from build123d import *

# Parameters (mm, degrees)
F1_DEPTH = 130
F2_W     = 50.8
F2_H     = 25.4
F3_DEPTH = 79.5
F4_W     = 12
F4_H     = 50.7057624385
F4_H_2   = 69.7820825055
F4_H_3   = 69.8881107867
F4_H_4   = 52.3517530859
F5_DEPTH = 47.4990536315


# Not quite as in the source:
# - ends of sketch curves that miss each other by under 0.0002 mm in the source are joined
# - a feature names something its author has since deleted; it is built from what else it names


with BuildPart() as f1:
    # F0 (on Right) → F1 (new body)
    with BuildSketch(Plane.YZ):
        with BuildLine():
            Line((62.1368927236, 13.271021442), (-57.8631072764, 13.271021442))
            Line((-57.8631072764, 13.271021442), (-57.8631072764, 7.697946392))
            Line((-57.8631072764, 7.697946392), (-56.4219683785, 7.6979366796))
            ThreePointArc((-56.4219683785, 7.6979366796), (-56.0194508606, 7.5356245361), (-55.8421445251, 7.1394791077))
            Line((-55.8421445251, 7.1394791077), (-54.3616227062, -32.302053608))
            ThreePointArc((-54.3616227062, -32.302053608), (-52.3630302548, -34.2270321895), (-50.3644378034, -32.302053608))
            Line((-50.3644378034, -32.302053608), (-48.8631072764, 7.697946392))
            ThreePointArc((-48.8631072764, 7.697946392), (-46.9131019002, 9.2535299318), (-44.9631072764, 7.6979329132))
            Line((-44.9631072764, 7.6979329132), (-43.4616227062, -32.302053608))
            ThreePointArc((-43.4616227062, -32.302053608), (-41.4630302548, -34.2270321895), (-39.4644378034, -32.302053608))
            Line((-39.4644378034, -32.302053608), (-37.9631072764, 7.697946392))
            ThreePointArc((-37.9631072764, 7.697946392), (-36.0131019002, 9.2535299318), (-34.0631072764, 7.6979329132))
            Line((-34.0631072764, 7.6979329132), (-32.5616227062, -32.302053608))
            ThreePointArc((-32.5616227062, -32.302053608), (-30.5630302548, -34.2270321895), (-28.5644378034, -32.302053608))
            Line((-28.5644378034, -32.302053608), (-27.0631072764, 7.697946392))
            ThreePointArc((-27.0631072764, 7.697946392), (-25.1131019002, 9.2535299318), (-23.1631072764, 7.6979329132))
            Line((-23.1631072764, 7.6979329132), (-21.6616227062, -32.302053608))
            ThreePointArc((-21.6616227062, -32.302053608), (-19.6630302548, -34.2270321895), (-17.6644378034, -32.302053608))
            Line((-17.6644378034, -32.302053608), (-16.1631072764, 7.697946392))
            ThreePointArc((-16.1631072764, 7.697946392), (-14.2131019002, 9.2535299318), (-12.2631072764, 7.6979329132))
            Line((-12.2631072764, 7.6979329132), (-10.7616227062, -32.302053608))
            ThreePointArc((-10.7616227062, -32.302053608), (-8.7630302548, -34.2270321895), (-6.7644378034, -32.302053608))
            Line((-6.7644378034, -32.302053608), (-5.2631072764, 7.697946392))
            ThreePointArc((-5.2631072764, 7.697946392), (-3.3131019002, 9.2535299318), (-1.3631072764, 7.6979329132))
            Line((-1.3631072764, 7.6979329132), (0.1383772938, -32.302053608))
            ThreePointArc((0.1383772938, -32.302053608), (2.1369697452, -34.2270321895), (4.1355621966, -32.302053608))
            Line((4.1355621966, -32.302053608), (5.6368927236, 7.697946392))
            ThreePointArc((5.6368927236, 7.697946392), (7.5868980998, 9.2535299318), (9.5368927236, 7.6979329132))
            Line((9.5368927236, 7.6979329132), (11.0383772938, -32.302053608))
            ThreePointArc((11.0383772938, -32.302053608), (13.0369697452, -34.2270321895), (15.0355621966, -32.302053608))
            Line((15.0355621966, -32.302053608), (16.5368927236, 7.697946392))
            ThreePointArc((16.5368927236, 7.697946392), (18.4868980998, 9.2535299318), (20.4368927236, 7.6979329132))
            Line((20.4368927236, 7.6979329132), (21.9383772938, -32.302053608))
            ThreePointArc((21.9383772938, -32.302053608), (23.9369697452, -34.2270321895), (25.9355621966, -32.302053608))
            Line((25.9355621966, -32.302053608), (27.4368927236, 7.697946392))
            ThreePointArc((27.4368927236, 7.697946392), (29.3868980998, 9.2535299318), (31.3368927236, 7.6979329132))
            Line((31.3368927236, 7.6979329132), (32.8383772938, -32.302053608))
            ThreePointArc((32.8383772938, -32.302053608), (34.8369697452, -34.2270321895), (36.8355621966, -32.302053608))
            Line((36.8355621966, -32.302053608), (38.3368927236, 7.697946392))
            ThreePointArc((38.3368927236, 7.697946392), (40.2868980998, 9.2535299318), (42.2368927236, 7.6979329132))
            Line((42.2368927236, 7.6979329132), (43.7383772938, -32.302053608))
            ThreePointArc((43.7383772938, -32.302053608), (45.7369697452, -34.2270321895), (47.7355621966, -32.302053608))
            Line((47.7355621966, -32.302053608), (49.2368927236, 7.697946392))
            ThreePointArc((49.2368927236, 7.697946392), (51.1868980998, 9.2535299318), (53.1368927236, 7.6979329132))
            Line((53.1368927236, 7.6979329132), (54.6383772938, -32.302053608))
            ThreePointArc((54.6383772938, -32.302053608), (56.6369697452, -34.2270321895), (58.6355621966, -32.302053608))
            Line((58.6355621966, -32.302053608), (60.11593154, 7.1394768706))
            ThreePointArc((60.11593154, 7.1394768706), (60.2932371534, 7.5356237596), (60.6957554774, 7.697946392))
            Line((60.6957554774, 7.697946392), (62.1368927236, 7.697946392))
            Line((62.1368927236, 7.697946392), (62.1368927236, 13.271021442))
        make_face()
    extrude(amount=F1_DEPTH)

    # F2 (on face) → F3 (cut)
    with BuildSketch(Plane.XY.offset(13.271021442)):
        with Locations((65, -45.1631072764)):
            Rectangle(F2_W, F2_H)
        with Locations((65, 49.4368927236)):
            Rectangle(F2_W, F2_H)
    extrude(amount=-F3_DEPTH, mode=Mode.SUBTRACT)

    # F4 (on face) → F5 (cut, through all)
    with BuildSketch(Plane.XY.offset(13.271021442)):
        with Locations((6, 36.890672449)):
            Rectangle(F4_W, F4_H)
        with Locations((6, -23.353250023)):
            Rectangle(F4_W, F4_H_2)
        with Locations((124, -23.955682084)):
            Rectangle(F4_W, F4_H_3)
        with Locations((124, 37.1642498523)):
            Rectangle(F4_W, F4_H_4)
    extrude(amount=-F5_DEPTH, mode=Mode.SUBTRACT)


solid = f1.part
CAD build for the part. Positions are in the model's coordinates, mm. A direction names the side the tool comes from. Round coordinates to 2 decimals unless told otherwise and drop trailing zeros. Write each loop counter-clockwise with the first axis right and the second up, starting at its lowest first coordinate (ties: lowest second). Pieces come first, ordered by that corner, then holes. Notation, with made-up numbers: M -4.5,67 L 37.5,67 A17 cw 37.5,83 Z; hole C 5,4.25 d8. An arc over 180 degrees is marked long. Put each result on its own line as item: value. Start each with the question number.
1) Pin check, flat tips, straight feed: pin 1 Ø1.2 at (x, y) = (105, 61.5) entering from -Z; pin 2 Ø12 at (x, z) = (80.5, -21) entering from +Y; pin 3 Ø23 at (x, z) = (74, -4) entering from -Y. Stop position of each tip, or through.
2) Saw through at A-A, the plane x = 56. Write the cut outline in (y, z), and give its area (3 significant figures).
3) Saw through at B-B, the plane z = -17. Count the separate pieces of the cut face and the enclosed holes in it, and give its area (3 significant figures).
4) Drill centre lines: probe 1 along X at (y, z) = (-48, 9.5); probe 2 along Z at (x, y) = (53, -20); probe 3 along Z at (x, y) = (35.5, -18.5). Where is each one in solid material? Low to high. Write a range as [from, to].
5) Pull direction X, two halves, no side cores. Call faces 1 (the flat face through (65, 36.737, -9)), 2 (the flat face through (118, 3, -5)), 3 (the flat face through (25.607, 48.476, -12.582)): pulls with the +X half, pulls with the -X half, needs draft (parallel to the pull), parting line crosses it, or undercut.
6) 3-axis set-ups, long thin cutter, end or side, ignore diameter. For faces 4 (the flat face through (104.007, 59.365, -12.857)), 5 (the flat face through (39.6, -43, -10)), 6 (the flat face through (90.4, 46, -5)), 7 (the flat face through (64.258, -16.924, -12.582)): which of +Z, -Z, +X, -X, +Y, -Y reach the whole face in a straight line?
Resolved:
1. pin 1: z = 7.7
1. pin 2: y = 36.74
1. pin 3: y = -32.46
2. outline: M -32.46,-32.85 A2 ccw -28.56,-32.3 L -27.06,7.7 A2 cw -23.16,7.7 L -21.66,-32.3 A2 ccw -17.66,-32.3 L -16.16,7.7 A2 cw -12.26,7.7 L -10.76,-32.3 A2 ccw -6.76,-32.3 L -5.26,7.7 A2 cw -1.36,7.7 L 0.14,-32.3 A2 ccw 4.14,-32.3 L 5.64,7.7 A2 cw 9.54,7.7 L 11.04,-32.3 A2 ccw 15.04,-32.3 L 16.54,7.7 A2 cw 20.44,7.7 L 21.94,-32.3 A2 ccw 25.94,-32.3 L 27.44,7.7 A2 cw 31.34,7.7 L 32.84,-32.3 A2 ccw 36.74,-32.85 L 36.74,13.27 L -32.46,13.27 Z
2. area: 1,870 mm²
3. separate pieces: 15
3. enclosed holes: 0
3. area: 4,890 mm²
4. probe 1: [12, 39.6], [90.4, 118]
4. probe 2: [-34.2, 13.27]
4. probe 3: [-33.85, 13.27]
5. face 1: undercut
5. face 2: pulls with the +X half
5. face 3: needs draft
6. face 4: -Z, +X, -X, +Y
6. face 5: +Z, -Z, -Y
6. face 6: +Z, -Z, +Y
6. face 7: -Z, +X, -X
